The model under review builds one solid part; all positions refer to its coordinate system, in mm. A direction names the side the tool comes from. Round coordinates to 2 decimals unless told otherwise and drop trailing zeros. Write each loop counter-clockwise with the first axis right and the second up, starting at its lowest first coordinate (ties: lowest second). Pieces come first, ordered by that corner, then holes.
Item 1: To check wall thickness, follow L1, parallel to Y at x = 0, z = 7.75 (3 decimals); L2, parallel to Z at x = -8, y = -2; L3, parallel to X at y = 13.25, z = -4.25. State the ranges of each line that lie inside material, in increasing order.
Item 2: Add section A-A (z = -11.25). Give the boundary of the cut face in (x, y).
Item 3: Machinability: for faces 4 (the face through (1.57, 3.02, -10.25)), 5 (the face through (5.32, 1.67, 8.31)), 6 (the face through (1.5, -1.5, 1)), which of the approach directions +Z, -Z, +X, -X, +Y, -Y give a long, thin tool a straight path to every point of the face, cutting with its end or side? Answer none if there is none.
Item 4: Add section B-B (z = -7.25). Give the boundary of the cut face in (x, y).
Item 5: Clearance check with flat-ended pins moving along their axes: pin 1 Ø1 at (x, y) = (0, -10.5) entering from -Z; pin 2 Ø1 at (x, z) = (11, -4) entering from +Y; pin 3 Ø8 at (y, z) = (-5.5, 1) entering from +X. State where each tip first meets the part, or that it passes through.
Item 6: Draft analysis for pull direction Z (two halves, no side actions). For faces 1 (the face through (-0.725, 0.228, -16.144)), 2 (the face through (0, 0, -17.28)), 3 (the face through (0, -4, 0)), state which applies: +Z half, -Z half, draft (parallel to the pull), parting line (faces both ways), or undercut.
```python
from build123d import *

# Parameters (mm, degrees)
SKETCH1_R           = 14.9
BOSS_EXTRUDE1_DEPTH = 10
FILLET1_R           = 5
SKETCH3_R           = 3.41
BOSS_EXTRUDE2_DEPTH = 1
SKETCH4_R           = 1.76
BOSS_EXTRUDE3_DEPTH = 5.9
SKETCH5_R           = 5.575
BOSS_EXTRUDE4_DEPTH = 2.86
SKETCH6_R           = 1.36
CUT_EXTRUDE1_DEPTH  = 2.86
SKETCH7_R           = 3.405
BOSS_EXTRUDE5_DEPTH = 0.5
SKETCH8_R           = 1.79
BOSS_EXTRUDE6_DEPTH = 1.92
SKETCH9_R           = 2.85
BOSS_EXTRUDE7_DEPTH = 1.12
SKETCH10_R          = 1.11
BOSS_EXTRUDE8_DEPTH = 1.5
BOSS_EXTRUDE8_TAPER = 5
SKETCH11_R          = 0.76
BOSS_EXTRUDE9_DEPTH = 2.24


with BuildPart() as part:
    # Sketch1 → Boss-Extrude1 (new body)
    with BuildSketch(Plane.XY):
        Circle(SKETCH1_R)
    extrude(amount=-BOSS_EXTRUDE1_DEPTH)

    # Fillet1
    fillet1_edges = [part.edges().sort_by_distance(p)[0] for p in [
        (-14.9, 0, 0),
        (-14.9, 0, -10),
    ]]
    fillet(fillet1_edges, radius=FILLET1_R - 0.0001)  # a hair under: the kernel refuses the full size

    # Sketch3 → Boss-Extrude2 (add)
    with BuildSketch(Plane.XY):
        Circle(SKETCH3_R)
    extrude(amount=BOSS_EXTRUDE2_DEPTH)

    # Sketch4 → Boss-Extrude3 (add)
    with BuildSketch(Plane.XY.offset(1)):
        Circle(SKETCH4_R)
    extrude(amount=BOSS_EXTRUDE3_DEPTH)

    # Sketch5 → Boss-Extrude4 (add)
    with BuildSketch(Plane.XY.offset(6.9)):
        Circle(SKETCH5_R)
    extrude(amount=BOSS_EXTRUDE4_DEPTH)

    # Sketch6 → Cut-Extrude1 (cut)
    with BuildSketch(Plane.XY.offset(9.76)):
        Circle(SKETCH6_R)
    extrude(amount=-CUT_EXTRUDE1_DEPTH, mode=Mode.SUBTRACT)

    # Sketch7 → Boss-Extrude5 (add)
    with BuildSketch(Plane(origin=(0, 0, -10), x_dir=(-1, 0, 0), z_dir=(0, 0, -1))):
        with Locations(Location((0, 0, 0), (0, 0, 180))):
            Circle(SKETCH7_R)
    extrude(amount=BOSS_EXTRUDE5_DEPTH)

    # Sketch8 → Boss-Extrude6 (add)
    with BuildSketch(Plane(origin=(0, 0, -10.5), x_dir=(-1, 0, 0), z_dir=(0, 0, -1))):
        Circle(SKETCH8_R)
    extrude(amount=BOSS_EXTRUDE6_DEPTH)

    # Sketch9 → Boss-Extrude7 (add)
    with BuildSketch(Plane(origin=(0, 0, -12.42), x_dir=(-1, 0, 0), z_dir=(0, 0, -1))):
        Circle(SKETCH9_R)
    extrude(amount=BOSS_EXTRUDE7_DEPTH)

    # Sketch10 → Boss-Extrude8 (add)
    with BuildSketch(Plane(origin=(0, 0, -13.54), x_dir=(-1, 0, 0), z_dir=(0, 0, -1))):
        Circle(SKETCH10_R)
    extrude(amount=BOSS_EXTRUDE8_DEPTH, taper=BOSS_EXTRUDE8_TAPER)

    # Sketch11 → Boss-Extrude9 (add)
    with BuildSketch(Plane(origin=(0, 0, -15.04), x_dir=(-1, 0, 0), z_dir=(0, 0, -1))):
        Circle(SKETCH11_R)
    extrude(amount=BOSS_EXTRUDE9_DEPTH)


solid = part.part
```
Numbers:
1. L1: y = -5.575 to -1.36, 1.36 to 5.575
1. L2: z = -10 to 0
1. L3: x = -6.69 to 6.69
2. outline: circle Ø3.58 at (0, 0)
3. face 4: -Z
3. face 5: +Z
3. face 6: none
4. outline: circle Ø28.73 at (0, 0)
5. pin 1: stops at z = -10
5. pin 2: stops at y = 10.45
5. pin 3: stops at x = 13.78
6. face 1: draft
6. face 2: -Z half
6. face 3: undercut
